from build123d import *

# Parameters (mm, degrees)
POCKET_DEPTH       = 201.453094
POLARPATTERN_COUNT = 3


with BuildPart() as part:
    # Sketch → Revolution (revolve)
    with BuildSketch(Plane.XZ):
        Polygon((2.7, 70), (11, 70), (11, 0), (10, -1), (10, -20), (5.964154, -20), (2.7, -13), align=None)
    revolve(axis=Axis((0, 0, 0), (0, 0, 1)))

    # Sketch001 (on DatumPlane) → Pocket (cut, through all)
    with BuildSketch(Plane(origin=(0, 0, -20), x_dir=(1, 0, 0), z_dir=(0, 1, 0))):
        with BuildLine():
            Line((0.5, -15), (0.5, 20))
            Line((0.5, 20), (-0.5, 20))
            Line((-0.5, 20), (-0.5, -15))
            ThreePointArc((-0.5, -15), (0, -15.5), (0.5, -15))
        make_face()
    pocket = extrude(amount=-POCKET_DEPTH, mode=Mode.SUBTRACT)

    # PolarPattern: Pocket ×3 about axis
    polarpattern_axis = Axis((0, 0, 0), (0, 0, 1))
    for i in range(1, POLARPATTERN_COUNT):
        add(pocket.rotate(polarpattern_axis, i * 360 / POLARPATTERN_COUNT), mode=Mode.SUBTRACT)


solid = part.part
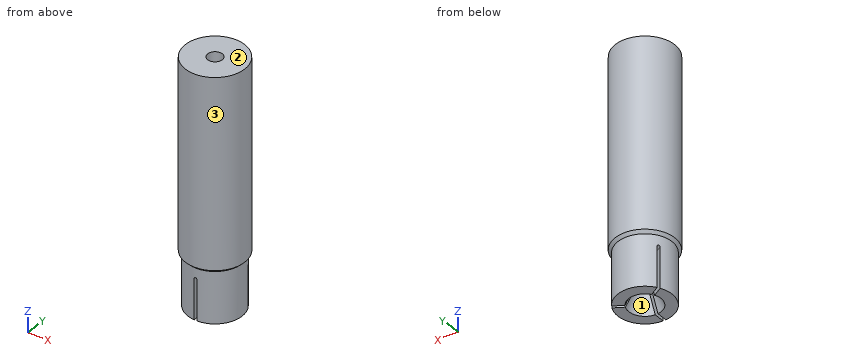
Verification items for the finished model (mm, model axes). Face numbers are marked on the shaded views. Give positions to 0.01 mm unless a question says otherwise; leave off trailing zeros. Loops run counter-clockwise (first coordinate to the right, second up) from the corner with the lowest first, then second, coordinate; pieces in that order, holes last. Notation, with made-up numbers: (79, -1) - (131, -1) arc R15 cw to (131, 18) - close; hole circle Ø8 at (56.25, 15.25). An arc over 180 degrees is marked (long way). Write each question's results on one line, items separated by ' | '.
1) Depth check by flat-ended pin: P1, Ø2, axis at x = -6, z = 24, coming from the +Y side; P2, Ø8, axis at y = -7.5, z = -11, coming from the -X side; P3, Ø3, axis at y = -7.5, z = 52, coming from the -X side; P4, Ø3, axis at x = 0, y = 0, coming from the +Z side. Enter the tip coordinate at first touch or a pass-through.
Solution:
P1: y = 9.8 | P2: x = -9.37 | P3: x = -9.22 | P4: through
2) Sectioned sample at A-A on y = 0. Record the boundary of the cut face in (x, z), plus the area to 3 significant figures.
Solution:
outline: (-11, 0) - (-10, -1) - (-10, -20) - (-5.96, -20) - (-2.7, -13) - (-2.7, 70) - (-11, 70) - close; (2.7, -13) - (5.96, -20) - (10, -20) - (10, -1) - (11, 0) - (11, 70) - (2.7, 70) - close | area: 1,430 mm2
3) Sectioned sample at B-B on z = 13.5. Record the boundary of the cut face in (x, y), plus the area to 3 significant figures.
Solution:
outline: circle Ø22 at (0, 0); hole circle Ø5.4 at (0, 0) | area: 357 mm2
4) Mould release check, pull along Y, two halves, no side actions. Record for the marked faces 1, 2 and 3: pulls with the +Y half, pulls with the -Y half, needs draft (parallel to the pull), parting line crosses it, or undercut.
Solution:
face 1: undercut | face 2: needs draft | face 3: parting line crosses it
5) Material ranges on L1, parallel to Y at x = 0, z = 13; L2, parallel to X at y = 2.5, z = -14; L3, parallel to X at y = -4.75, z = -9, recorded low to high. Write a range as from..to.
Solution:
L1: -11..-2.7, 2.7..11 | L2: -9.68..-5.33, -3.33..-1.94, 1.94..3.33, 5.33..9.68 | L3: -8.8..-0.5, 0.5..8.8
